Part model, mm, in its own coordinate system. A direction names the side the tool comes from. Coordinates: 2 decimals unless noted, no trailing zeros. Order: outer loops, then holes, each group sorted by start corner. A loop starts at its lowest first (then second) coordinate and runs counter-clockwise, first axis right, second up. Notation, with made-up numbers: (86.5, 65.25) - (121.5, 65.25) arc R14 cw to (121.5, 81.25) - close; hole circle Ø10 at (15.5, -18.5). An arc over 180 degrees is marked (long way). Use a Markdown table: item, result. Add a question column.
1) Drop flat-ended pins along their axis: P1, Ø1.5, axis at x = -2, y = 30, coming from the -Z side; P2, Ø4, axis at x = 0, z = 0, coming from the -Y side; P3, Ø1.5, axis at x = -3.5, y = 55, coming from the -Z side. Give the stop position or say it passes through.
2) Wall check: L1, parallel to Z at x = 0, y = 8.25; L2, parallel to X at y = 107.75, z = 0; L3, parallel to Y at x = -0.75, z = 1.5. Give the ranges that are in metal, low to high. Write a range as [from, to].
3) Saw through at C-C on y = 49.5. List the corners of the cut face in (x, z), then the cut area to 3 significant figures.
4) Saw through at B-B on z = 0. List the corners of the cut face in (x, y), then the cut area to 3 significant figures.
5) Saw through at A-A on y = 16. List the corners of the cut face in (x, z), then the cut area to 3 significant figures.
6) Two-plate mould, pull along X, no slides. Class faces 1 (the face through (-6.35, 56, 0)), 2 (the face through (3.131, 55.724, -5.525)), 3 (the face through (0, 25.4, 0)): +X half, -X half, draft (parallel to the pull), parting line (faces both ways), or undercut.
7) Tool access for faces 4 (the face through (-0.748, 12.878, -2.374)), 5 (the face through (3.219, 55.724, 5.474)), 6 (the face through (-0.748, 100.152, 2.374)): list every direction of +Z, -Z, +X, -X, +Y, -Y with a clear straight run to the whole face (end or side of a thin tool).
8) Saw through at D-D on x = 1. List the corners of the cut face in (y, z).
Autodesk Inventor part; units mm, degrees
ref_plane "YZ Plane" through (0, 0, 0) normal (1, 0, 0) x (0, 1, 0)
ref_plane "XZ Plane" through (0, 0, 0) normal (0, 1, 0) x (-1, 0, 0)
ref_plane "XY Plane" through (0, 0, 0) normal (0, 0, 1) x (1, 0, 0)
sketch "Sketch1" plane through (0, 0, 0) normal (0, 1, 0) x (-1, 0, 0)
  line L0 (6.35, -3.6662) -> (0, -7.3323)
  line L1 (0, -7.3323) -> (-6.35, -3.6662)
  line L2 (-6.35, -3.6662) -> (-6.35, 3.6662)
  line L3 (-6.35, 3.6662) -> (0, 7.3323)
  line L4 (0, 7.3323) -> (6.35, 3.6662)
  line L5 (6.35, 3.6662) -> (6.35, -3.6662)
  point P0 (0, 0)
  point P1 (0, 0)
  point P2 (0, 0)
  dimension "d0" = 12.7
extrude "Extrusion1" add sketch "Sketch1" along normal blind 113.03
sketch "Sketch2" plane through (0, 113.03, 0) normal (0, 1, 0) x (1, 0, 0)
  point P0 (0, 0)
  point P1 (0, 0)
hole "Hole1" at (0, 113.03, 0) direction (0, -1, 0) diameter 4.9784 depth 25.4
sketch "Sketch3" plane through (0, 0, 0) normal (0, -1, 0) x (1, 0, 0)
  point P0 (0, 0)
  point P1 (0, 0)
hole "Hole2" at (0, 0, 0) direction (0, 1, 0) diameter 4.9784 depth 25.4
properties part number "ELEV_041_HEXSHAFT4" material "Aluminum 6061"
Results are:
| question | item | result |
|---|---|---|
| 1 | P1 | z = -6.61 |
| 1 | P2 | y = 25.4 |
| 1 | P3 | z = -5.74 |
| 2 | L1 | [-7.33, -2.49], [2.49, 7.33] |
| 2 | L2 | [-6.35, -2.49], [2.49, 6.35] |
| 2 | L3 | [25.4, 87.63] |
| 3 | outline | (-6.35, -3.67) - (0, -7.33) - (6.35, -3.67) - (6.35, 3.67) - (0, 7.33) - (-6.35, 3.67) - close |
| 3 | area | 140 mm2 |
| 4 | outline | (-6.35, 0) - (-2.49, 0) - (-2.49, 25.4) - (2.49, 25.4) - (2.49, 0) - (6.35, 0) - (6.35, 113.03) - (2.49, 113.03) - (2.49, 87.63) - (-2.49, 87.63) - (-2.49, 113.03) - (-6.35, 113.03) - close |
| 4 | area | 1,180 mm2 |
| 5 | outline | (-6.35, -3.67) - (0, -7.33) - (6.35, -3.67) - (6.35, 3.67) - (0, 7.33) - (-6.35, 3.67) - close; hole circle Ø4.98 at (0, 0) |
| 5 | area | 120 mm2 |
| 6 | face 1 | -X half |
| 6 | face 2 | +X half |
| 6 | face 3 | undercut |
| 7 | face 4 | -Y |
| 7 | face 5 | +Z, +X, +Y, -Y |
| 7 | face 6 | +Y |
| 8 | outline | (0, -6.75) - (113.03, -6.75) - (113.03, -2.28) - (87.63, -2.28) - (87.63, 2.28) - (113.03, 2.28) - (113.03, 6.75) - (0, 6.75) - (0, 2.28) - (25.4, 2.28) - (25.4, -2.28) - (0, -2.28) - close |
